Read the model definition and answer for the solid it produces. Units are mm, in the model's axes. A direction names the side the tool comes from. Give positions to 0.01 mm unless a question says otherwise; leave off trailing zeros. Order: outer loops, then holes, each group sorted by start corner. A loop starts at its lowest first (then second) coordinate and runs counter-clockwise, first axis right, second up. Notation, with made-up numbers: M 30,27.25 L 61,27.25 A28 cw 61,53.25 Z; hole C 21,4 d1. An arc over 180 degrees is marked long. One line per item, written item: value.
from build123d import *

# Parameters (mm, degrees)
F1_DEPTH = 6
F4_T     = 1.8
F6_DEPTH = 7.8


with BuildPart() as f1:
    # F0 (on Top) → F1 (new body)
    with BuildSketch(Plane.XY):
        with BuildLine():
            Line((12.95, 16.7), (-12.95, 16.7))
            ThreePointArc((-12.95, 16.7), (-16.4855339059, 15.2355339059), (-17.95, 11.7))
            Line((-17.95, 11.7), (-17.95, -11.7))
            ThreePointArc((-17.95, -11.7), (-16.4855339059, -15.2355339059), (-12.95, -16.7))
            Line((-12.95, -16.7), (12.95, -16.7))
            ThreePointArc((12.95, -16.7), (16.4855339059, -15.2355339059), (17.95, -11.7))
            Line((17.95, -11.7), (17.95, 11.7))
            ThreePointArc((17.95, 11.7), (16.4855339059, 15.2355339059), (12.95, 16.7))
        make_face()
    extrude(amount=F1_DEPTH)

    # F2 (on Front) → F3 (revolve)
    with BuildSketch(Plane.XZ):
        with BuildLine():
            Line((0, 9.8057864234), (0, 6))
            Line((0, 6), (12.95, 6))
            Line((12.95, 6), (14.9687874717, 6))
            ThreePointArc((14.9687874717, 6), (7.7225094476, 8.8394416898), (0, 9.8057864234))
        make_face()
    revolve(axis=Axis((0, 0, 7.9028932117), (0, 0, 1)))

    # F4
    f4_openings = [f1.faces().sort_by_distance(p)[0] for p in [
        (0, 0, 0),
    ]]
    offset(amount=F4_T, openings=f4_openings, kind=Kind.INTERSECTION)

    # F5 (on face) → F6 (join, through all)
    with BuildSketch(Plane.XY.offset(7.8)):
        with BuildLine():
            ThreePointArc((19.75, 4.0565560225), (22.4501669969, 1.9970193201), (23.4744745018, -1.2407866307))
            ThreePointArc((23.4744745018, -1.2407866307), (22.4501669969, -4.4785925814), (19.75, -6.5381292838))
            Line((19.75, -6.5381292838), (19.75, -8.942287067))
            ThreePointArc((19.75, -8.942287067), (24.0922338374, -6.1310158755), (25.7786200161, -1.2407866307))
            ThreePointArc((25.7786200161, -1.2407866307), (24.0922338374, 3.6494426142), (19.75, 6.4607138057))
            Line((19.75, 6.4607138057), (19.75, 4.0565560225))
        make_face()
    extrude(amount=-F6_DEPTH)


solid = f1.part
1) Find section C-C, the plane x = -1.5. Write down the section's boundary in (y, z), plus the area to 3 significant figures.
Reported:
outline: M -18.5,0 L -16.7,0 L -16.7,6 L -14.89,6 A31.3 cw 14.89,6 L 16.7,6 L 16.7,0 L 18.5,0 L 18.5,7.8 L 15.35,7.8 A33.11 ccw -15.35,7.8 L -18.5,7.8 Z
area: 90.5 mm^2
2) Which of the six approach directions +Z, -Z, +X, -X, +Y, -Y give full straight-line access (tool end or side, diameter ignored) to faces 1 (the face through (3, -16, 7.8)), 2 (the face through (19.75, -1, 4)), 3 (the face through (-17.95, 0, 3)), 4 (the face through (19.75, -10, 4))?
Reported:
face 1: +Z
face 2: +Z, -Z
face 3: -Z
face 4: +Z, -Z, +X, -Y
3) Consider probe 1 along X at (y, z) = (-10, 4.25); probe 2 along X at (y, z) = (1, 2); probe 3 along Y at (x, z) = (-11, 5). Determine where each line is inside the solid, lowest interval first.
Reported:
probe 1: x = -19.75 to -17.95, 17.95 to 19.75
probe 2: x = -19.75 to -17.95, 17.95 to 19.75, 23.01 to 25.46
probe 3: y = -18.5 to -16.7, 16.7 to 18.5
4) Find section A-A, the plane z = 3.25. Write down the section's boundary in (x, y).
Reported:
outline: M -19.75,-11.7 A6.8 ccw -12.95,-18.5 L 12.95,-18.5 A6.8 ccw 19.75,-11.7 L 19.75,-8.94 A7.93 ccw 19.75,6.46 L 19.75,11.7 A6.8 ccw 12.95,18.5 L -12.95,18.5 A6.8 ccw -19.75,11.7 Z; hole M -17.95,-11.7 A5 ccw -12.95,-16.7 L 12.95,-16.7 A5 ccw 17.95,-11.7 L 17.95,11.7 A5 ccw 12.95,16.7 L -12.95,16.7 A5 ccw -17.95,11.7 Z; hole M 19.75,-6.54 A5.63 ccw 19.75,4.06 Z
5) Each of these flat-tipped pins is pushed along its axis until it touches: pin 1 Ø1.6 at (y, z) = (9.5, 5.5) entering from +X; pin 2 Ø6.5 at (y, z) = (-1.5, 2) entering from +X; pin 3 Ø2.5 at (y, z) = (1.5, 4) entering from +X; pin 4 Ø8 at (x, y) = (20, 8.5) entering from +Z. Where does it stop, or does it pass through?
Reported:
pin 1: stops at x = 19.75
pin 2: stops at x = 25.78
pin 3: stops at x = 25.64
pin 4: stops at z = 7.8
6) Determine the mould class of faces 5 (the face through (0, -18.5, 4)), 6 (the face through (0, 16.7, 3)), 7 (the face through (16.45, -15.27, 2.96)), 8 (the face through (0, 18.5, 4)) for opening direction Y: +Y half, -Y half, draft (parallel to the pull), parting line (faces both ways), or undercut.
Reported:
face 5: -Y half
face 6: undercut
face 7: undercut
face 8: +Y half
7) Find section D-D, the plane z = 6.5. Write down the section's boundary in (x, y), plus the area to 3 significant figures.
Reported:
outline: M -19.75,-11.7 A6.8 ccw -12.95,-18.5 L 12.95,-18.5 A6.8 ccw 19.75,-11.7 L 19.75,-8.94 A7.93 ccw 19.75,6.46 L 19.75,11.7 A6.8 ccw 12.95,18.5 L -12.95,18.5 A6.8 ccw -19.75,11.7 Z; hole C 0,0 d28.02; hole M 19.75,-6.54 A5.63 ccw 19.75,4.06 Z
area: 845 mm^2
8) Find section B-B, the plane y = 3. Write down the section's boundary in (x, z) (3 decimals).
Reported:
outline: M -19.75,0 L -17.95,0 L -17.95,6 L -14.665,6 A31.196 cw 14.665,6 L 17.95,6 L 17.95,0 L 19.75,0 L 19.75,7.8 L 15.125,7.8 A33.004 ccw -15.125,7.8 L -19.75,7.8 Z; M 21.547,0 L 24.55,0 L 24.55,7.8 L 21.547,7.8 Z
